from build123d import *

# Parameters (mm, degrees)
BOSS_EXTRUDE1_DEPTH = 800
FILLET1_R           = 3


with BuildPart() as part:
    # Sketch2 → Boss-Extrude1 (new body)
    with BuildSketch(Plane(origin=(0, 0, 0), x_dir=(1, 0, 0), z_dir=(0, 1, 0))):
        with BuildLine():
            Line((38, 12.187104498), (38, -17.812895502))
            ThreePointArc((38, -17.812895502), (34.80462792, -16.696369068), (33, -13.832743381))
            Line((33, -13.832743381), (33, 7.187104498))
            Line((33, 7.187104498), (-33, 7.187104498))
            Line((-33, 7.187104498), (-33, -13.832743381))
            ThreePointArc((-33, -13.832743381), (-34.80462792, -16.696369068), (-38, -17.812895502))
            Line((-38, -17.812895502), (-38, 12.187104498))
            Line((-38, 12.187104498), (38, 12.187104498))
        make_face()
    extrude(amount=BOSS_EXTRUDE1_DEPTH)

    # Fillet1
    fillet1_edges = [part.edges().sort_by_distance(p)[0] for p in [
        (38, 400, -12.187104498),
        (33, 400, -7.187104498),
        (-33, 400, -7.187104498),
        (-38, 400, -12.187104498),
    ]]
    fillet(fillet1_edges, radius=FILLET1_R)


solid = part.part
Geometry: final body of the model. Coordinates: model frame, mm. A direction names the side the tool comes from. Coordinates: 2 decimals unless noted, no trailing zeros. Order: outer loops, then holes, each group sorted by start corner. A loop starts at its lowest first (then second) coordinate and runs counter-clockwise, first axis right, second up. Notation, with made-up numbers: M -28.75,-30.75 L -19.75,-30.75 A22 ccw -19.75,-21.75 Z; hole C 39,27 d8. An arc over 180 degrees is marked long. One line per question, with ' | ' between items. Start each with the question number.
Item 1: Cut plane C-C, the plane x = 0.5. Return the cut outline in (y, z), then the cut area to 3 significant figures.
Item 2: Cut plane A-A, the plane z = 5. Return the cut outline in (x, y).
Item 3: Pin query (flat end, axial travel): pin 1 Ø10 at (x, y) = (-9.5, 640) entering from +Z; pin 2 Ø10 at (x, z) = (-23.5, 2.5) entering from -Y. Return the tip coordinate at first contact, or that it passes through.
Item 4: Draft query along X for faces 1 (the flat face through (38, 394, 4)), 2 (the flat face through (0, 394, -12.187)), 3 (the flat face through (0, 394, -7.187)), 4 (the flat face through (33, 394, 5)). Return one class per face: released by +X, released by -X, zero draft, split by the parting line, or undercut.
Item 5: Cut plane B-B, the plane y = 72.5. Return the cut outline in (x, z).
Item 6: Ray query, probe 1 along X at (y, z) = (746.5, 9); probe 2 along X at (y, z) = (180.5, -10); probe 3 along Z at (x, y) = (25, 758). Return the intervals inside material, ascending. Write a range as [from, to].
Item 7: Set-up query: faces 5 (the flat face through (-33, 394, 5)), 6 (the flat face through (-38, 394, 5)). Return all of +Z, -Z, +X, -X, +Y, -Y with unobstructed straight access to the full face (end or side cutting, diameter ignored); none if empty.
A:
1) outline: M 0,-12.19 L 800,-12.19 L 800,-7.19 L 0,-7.19 Z | area: 4,000 mm2
2) outline: M -38,0 L -33,0 L -33,800 L -38,800 Z; M 33,0 L 38,0 L 38,800 L 33,800 Z
3) pin 1: stops at z = -7.19 | pin 2: passes through
4) face 1: released by +X | face 2: zero draft | face 3: undercut | face 4: undercut
5) outline: M -38,-9.19 A3 ccw -35,-12.19 L 35,-12.19 A3 ccw 38,-9.19 L 38,17.81 A5.13 ccw 33,13.83 L 33,-4.19 A3 cw 30,-7.19 L -30,-7.19 A3 cw -33,-4.19 L -33,13.83 A5.13 ccw -38,17.81 Z
6) probe 1: x = [-38, -33], [33, 38] | probe 2: x = [-37.89, 37.89] | probe 3: z = [-12.19, -7.19]
7) face 5: +Z, +Y, -Y | face 6: +Z, -Z, -X, +Y, -Y
